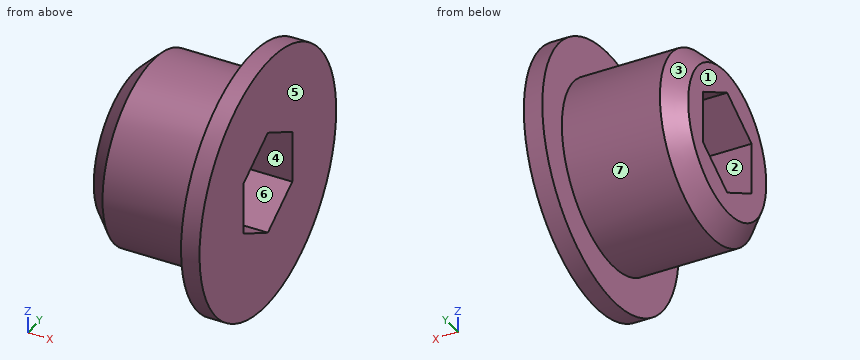
```python
from build123d import *

# Parameters (mm, degrees)
SKETCH_1_R      = 5
EXTRUDE_1_DEPTH = 6.3
SKETCH_2_R      = 7
EXTRUDE_2_DEPTH = 1
CHAMFER_1_SIZE  = 1


with BuildPart() as part:
    # 草图1 → 凸台-拉伸1 (new body)
    with BuildSketch(Plane(origin=(0, 0, 0), x_dir=(0, 0, -1), z_dir=(1, 0, 0))):
        Circle(SKETCH_1_R)
        Polygon((2.886751346, 0), (1.443375673, 2.5), (-1.443375673, 2.5), (-2.886751346, 0), (-1.443375673, -2.5), (1.443375673, -2.5), align=None, mode=Mode.SUBTRACT)
    extrude(amount=EXTRUDE_1_DEPTH)

    # 草图2 → 凸台-拉伸2 (add)
    with BuildSketch(Plane(origin=(6.3, 0, 0), x_dir=(0, 0, -1), z_dir=(1, 0, 0))):
        Circle(SKETCH_2_R)
        Polygon((2.886751346, 0), (1.443375673, 2.5), (-1.443375673, 2.5), (-2.886751346, 0), (-1.443375673, -2.5), (1.443375673, -2.5), align=None, mode=Mode.SUBTRACT)
    extrude(amount=EXTRUDE_2_DEPTH)

    # 倒角1
    chamfer_1_edges = [part.edges().sort_by_distance(p)[0] for p in [
        (0, 0, 5),
    ]]
    chamfer(chamfer_1_edges, length=CHAMFER_1_SIZE)


solid = part.part
```
The model under review builds one solid part; all positions refer to its coordinate system, in mm. Face numbers are marked on the shaded views. A direction names the side the tool comes from. Round coordinates to 2 decimals unless told otherwise and drop trailing zeros. Order: outer loops, then holes, each group sorted by start corner. A loop starts at its lowest first (then second) coordinate and runs counter-clockwise, first axis right, second up.
(1) For P1, Ø1, axis at y = 4.5, z = -5.5, coming from the +X side; P2, Ø2, axis at x = 2.5, y = -3.5, coming from the +Z side; P3, Ø1.5, axis at x = 4, z = -5, coming from the -Y side; P4, Ø3, axis at x = 4, z = 0.5, coming from the -Y side, all flat-tipped, find the tip position at first contact; note any pin that passes through.
Working result:
P1: stops at x = 7.3
P2: stops at z = 4.33
P3: stops at y = -2.63
P4: stops at y = -5
(2) Mouldability with a two-part tool opening along Z and no side actions: class the marked faces 1, 2, 3 and 4 as released by +Z, released by -Z, zero draft, split by the parting line, or undercut.
Working result:
face 1: zero draft
face 2: undercut
face 3: split by the parting line
face 4: undercut
(3) Take a section at C-C, the plane y = 6. State the section outline as (x, z) points, plus the area to 3 significant figures.
Working result:
outline: (6.3, -3.61) - (7.3, -3.61) - (7.3, 3.61) - (6.3, 3.61) - close
area: 7.21 mm2
(4) Wall thickness on L1, parallel to X at y = -1.5, z = 5; L2, parallel to Y at x = 2.75, z = 3; L3, parallel to Y at x = 3.75, z = -1.25: over which ranges is each line inside the solid? List them lowest first.
Working result:
L1: x = 6.3 to 7.3
L2: y = -4 to 4
L3: y = -4.84 to -2.5, 2.5 to 4.84
(5) Take a section at A-A, the plane z = 0. State the section outline as (x, y) points, plus the area to 3 significant figures.
Working result:
outline: (0, -4) - (1, -5) - (6.3, -5) - (6.3, -7) - (7.3, -7) - (7.3, -2.5) - (0, -2.5) - close; (0, 2.5) - (7.3, 2.5) - (7.3, 7) - (6.3, 7) - (6.3, 5) - (1, 5) - (0, 4) - close
area: 39.5 mm2
(6) Take a section at B-B, the plane x = 2. State the section outline as (y, z) points.
Working result:
outline: circle Ø10 at (0, 0); hole (-2.5, -1.44) - (0, -2.89) - (2.5, -1.44) - (2.5, 1.44) - (0, 2.89) - (-2.5, 1.44) - close
(7) Tool access review of the marked faces 5, 6 and 7: name each direction out of +Z, -Z, +X, -X, +Y, -Y from which nothing blocks a thin tool from reaching the whole face with its end or side.
Working result:
face 5: +Z, -Z, +X, +Y, -Y
face 6: +X, -X
face 7: -X
